Design review of the part built by this model. Coordinates are the model's own, in mm. Face numbers are marked on the shaded views. A direction names the side the tool comes from. Give positions to 0.01 mm unless a question says otherwise; leave off trailing zeros. Loops run counter-clockwise (first coordinate to the right, second up) from the corner with the lowest first, then second, coordinate; pieces in that order, holes last. Notation, with made-up numbers: (37, 82) - (43, 82) arc R16 ccw to (43, 113) - close; hole circle Ø7 at (13, 6). An arc over 180 degrees is marked (long way). Write each question's results on one line, items separated by ' | '.
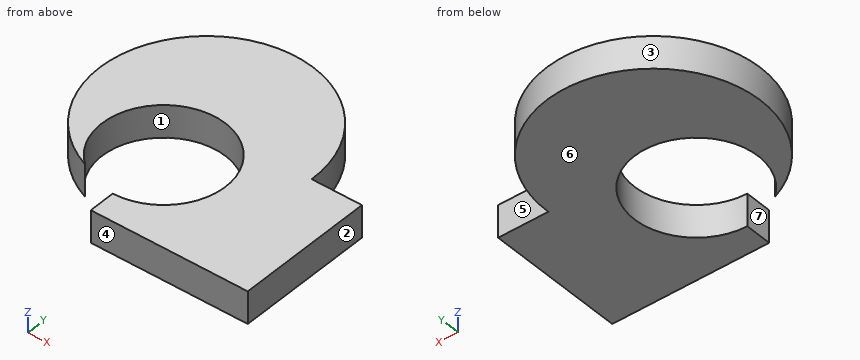
```python
from build123d import *

# Parameters (mm, degrees)
F0_W     = 24.360565
F0_H     = 21.410812
F1_DEPTH = 5
F2_R     = 16.571277
F3_DEPTH = 5
F4_R     = 9.566685
F5_DEPTH = 6


with BuildPart() as f1:
    # F0 (on Top) → F1 (new body)
    with BuildSketch(Plane.XY):
        with Locations((12.180282, -10.705406)):
            Rectangle(F0_W, F0_H)
    extrude(amount=F1_DEPTH)

    # F2 (on Top) → F3 (join)
    with BuildSketch(Plane.XY):
        with Locations((0, 0.314523)):
            Circle(F2_R)
    extrude(amount=F3_DEPTH)

    # F4 (on face) → F5 (cut)
    with BuildSketch(Plane.XY.offset(5)):
        with Locations((0, -7.725909)):
            Circle(F4_R)
    extrude(amount=-F5_DEPTH, mode=Mode.SUBTRACT)


solid = f1.part
```
Item 1: We need section B-B on y = 14. Give the boundary of the cut face in (x, z), then the cut area to 3 significant figures.
Output values:
outline: (-9.34, 0) - (9.34, 0) - (9.34, 5) - (-9.34, 5) - close | area: 93.4 mm²
Item 2: Tool access review of the marked faces 5, 6 and 7: name each direction out of +Z, -Z, +X, -X, +Y, -Y from which nothing blocks a thin tool from reaching the whole face with its end or side.
Output values:
face 5: +Z, -Z, +X, +Y | face 6: -Z, +X, -X, +Y, -Y | face 7: +Z, -Z, -X, -Y
Item 3: Draft analysis for pull direction Y (two halves, no side actions). For the marked faces 1, 2, 3 and 4, state which applies: +Y half, -Y half, draft (parallel to the pull), parting line (faces both ways), or undercut.
Output values:
face 1: undercut | face 2: draft | face 3: parting line | face 4: -Y half
Item 4: We need section C-C on y = 7.5. Give the boundary of the cut face in (x, z), then the cut area to 3 significant figures.
Output values:
outline: (-14.93, 0) - (14.93, 0) - (14.93, 5) - (-14.93, 5) - close | area: 149 mm²
Item 5: Wall thickness on probe 1 along X at (y, z) = (-3.5, 3.7); probe 2 along Y at (x, z) = (20, 4.5); probe 3 along Y at (x, z) = (2, 4.7): over which ranges is each line inside the solid? List them lowest first.
Output values:
probe 1: x = -16.13 to -8.58, 8.58 to 24.36 | probe 2: y = -21.41 to 0 | probe 3: y = -21.41 to -17.08, 1.63 to 16.76
Item 6: Clearance check with a flat-ended pin moving along its axis: P1, Ø1, axis at x = -4.5, z = 2, coming from the -Y side. State where the tip first meets the part, or that it passes through.
Output values:
P1: stops at y = 0.43
Item 7: We need section A-A on z = 1.95. Give the boundary of the cut face in (x, y), then the cut area to 3 significant figures.
Output values:
outline: (-6.11, -15.09) arc R9.57 cw (long way) to (0, -17.29) - (0, -21.41) - (24.36, -21.41) - (24.36, 0) - (16.57, 0) arc R16.57 ccw (long way) to start | area: 891 mm²
